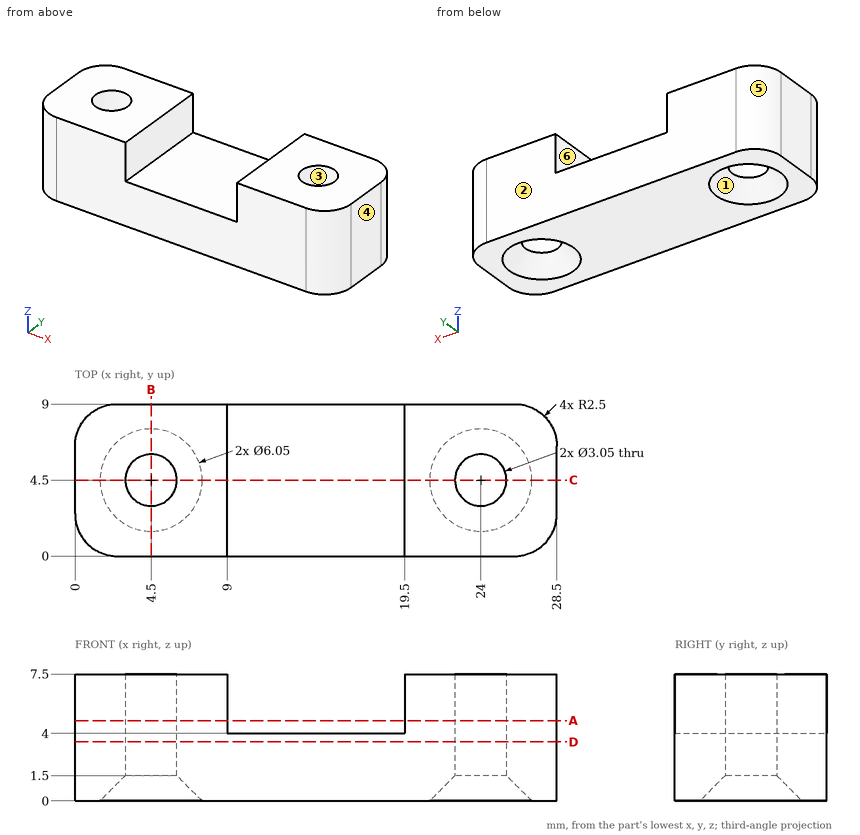
Geometry: see drawing. Coordinates: mm, zero at the bounding-box minimum. A direction names the side the tool comes from. Coordinates: 2 decimals unless noted, no trailing zeros. Loops run counter-clockwise (first coordinate to the right, second up) from the corner with the lowest first, then second, coordinate; pieces in that order, holes last. Notation, with made-up numbers: (72, 20.25) - (99, 20.25) arc R33 ccw to (99, 56.25) - close; hole circle Ø6 at (65.5, -32.5). An arc over 180 degrees is marked (long way). Return JSON: item names as keys, results as strings.
Q1. Material intervals for line 1 along X through (y, z) = (3.5, 4.75); line 2 along Y through (x, z) = (24, 5) (3 decimals); line 3 along X through (y, z) = (3.25, 1), sorted ascending.
Results:
{"line 1": "0 to 3.35, 5.65 to 9, 19.5 to 22.85, 25.15 to 28.5", "line 2": "0 to 2.975, 6.025 to 9", "line 3": "0 to 2.91, 6.09 to 22.41, 25.59 to 28.5"}
Q2. Section C-C, the plane y = 4.5. Return loops of the section in (x, z) (3 decimals).
Results:
{"outline": "(0, 0) - (1.475, 0) - (2.975, 1.5) - (2.975, 7.5) - (0, 7.5) - close; (6.025, 1.5) - (7.525, 0) - (20.975, 0) - (22.475, 1.5) - (22.475, 7.5) - (19.5, 7.5) - (19.5, 4) - (9, 4) - (9, 7.5) - (6.025, 7.5) - close; (25.525, 1.5) - (27.025, 0) - (28.5, 0) - (28.5, 7.5) - (25.525, 7.5) - close"}
Q3. Contact query for flat-ended pins moving along their axis: P1, Ø1.5, axis at x = 13.5, y = 4.5, coming from the +Z side; P2, Ø4, axis at x = 24, y = 4.5, coming from the -Z side (3 decimals). Output: stop coordinate, or through.
Results:
{"P1": "z = 4", "P2": "z = 1.025"}
Q4. Section A-A, the plane z = 4.75. Return loops of the section in (x, y) (3 decimals), plus the area to 3 significant figures.
Results:
{"outline": "(0, 2.5) arc R2.5 ccw to (2.5, 0) - (9, 0) - (9, 9) - (2.5, 9) arc R2.5 ccw to (0, 6.5) - close; (19.5, 0) - (26, 0) arc R2.5 ccw to (28.5, 2.5) - (28.5, 6.5) arc R2.5 ccw to (26, 9) - (19.5, 9) - close; hole circle Ø3.05 at (4.5, 4.5); hole circle Ø3.05 at (24, 4.5)", "area": "142 mm2"}
Q5. Access query for the marked faces 5 and 6. Directions: +Z, -Z, +X, -X, +Y, -Y. A direction counts if a zero-diameter tool reaches every point of the face in a straight line with its end or side. Return the directions, or none.
Results:
{"face 5": "+Z, -Z, -X, +Y", "face 6": "+Z, +Y, -Y"}
Q6. Section D-D, the plane z = 3.5. Return loops of the section in (x, y) (3 decimals), plus the area to 3 significant figures.
Results:
{"outline": "(0, 2.5) arc R2.5 ccw to (2.5, 0) - (26, 0) arc R2.5 ccw to (28.5, 2.5) - (28.5, 6.5) arc R2.5 ccw to (26, 9) - (2.5, 9) arc R2.5 ccw to (0, 6.5) - close; hole circle Ø3.05 at (4.5, 4.5); hole circle Ø3.05 at (24, 4.5)", "area": "237 mm2"}
Q7. Mould query, pull axis Y, two halves, no side actions, for the marked faces 1, 2, 3 and 4. Classes: released by +Y, released by -Y, zero draft, split by the parting line, or undercut.
Results:
{"face 1": "undercut", "face 2": "released by +Y", "face 3": "undercut", "face 4": "zero draft"}
Q8. Section B-B, the plane x = 4.5. Return loops of the section in (y, z) (3 decimals).
Results:
{"outline": "(0, 0) - (1.475, 0) - (2.975, 1.5) - (2.975, 7.5) - (0, 7.5) - close; (6.025, 1.5) - (7.525, 0) - (9, 0) - (9, 7.5) - (6.025, 7.5) - close"}
